For this review, take the finished solid that the model builds, in its own axes (mm). A direction names the side the tool comes from. Coordinates: 2 decimals unless noted, no trailing zeros. Loops run counter-clockwise (first coordinate to the right, second up) from the corner with the lowest first, then second, coordinate; pieces in that order, holes last. Notation, with made-up numbers: M -33,13 L -5,13 A21 cw -5,21 Z; hole C 51.5,64.25 d3. An arc over 180 degrees is marked long. Answer as a JSON object with one key per item and string values. Group by question number.
Item 1: Add section C-C (z = 16). State the section outline as (x, y) points (3 decimals).
Item 2: Add section A-A (x = 0). State the section outline as (y, z) points (1 decimal).
Item 3: Add section B-B (y = -0.5). State the section outline as (x, z) points (1 decimal).
Item 4: Wall thickness on L1, parallel to Y at x = 0, z = 14.3 (3 decimals); L2, parallel to Y at x = 0, z = 18.6 (3 decimals); L3, parallel to X at y = -2.25, z = 18.25: over which ranges is each line inside the solid? List them lowest first. Write a range as from..to.
Item 5: Add section D-D (y = -2). State the section outline as (x, z) points (1 decimal), then the cut area to 3 significant figures.
Item 6: Tool access review of faces 4 (the face through (2.731, 4.283, 18.545)), 5 (the face through (5.605, -0.098, 12.833)): name each direction out of +Z, -Z, +X, -X, +Y, -Y from which nothing blocks a thin tool from reaching the whole face with its end or side.
Item 7: Mouldability with a two-part tool opening along Y and no side actions: class faces 1 (the face through (0, -6.985, 16)), 2 (the face through (2, -2, 17.59)), 3 (the face through (-7.1, -0.1, 15.23)) as +Y half, -Y half, draft (parallel to the pull), parting line (faces both ways), or undercut.
Item 8: Insertion check: pin 1 (1.5 mm diameter, centred on y = -1.5, z = 18.5, fed in from +X); pin 2 (8 mm diameter, centred on x = -2, y = 0.5, fed in from +Z); pin 3 (5 mm diameter, centred on x = 1, y = 1.5, fed in from +Z). Each pin has a flat end and moves straight along its axis. Give the tip position at first contact, or say it passes through.
from build123d import *

# Parameters (mm, degrees)
F1_DEPTH = 6.985
F4_R     = 5.08
F5_DEPTH = 2.413
F6_R     = 2.54
F7_DEPTH = 5.2171329375
F8_R     = 1.27


with BuildPart() as f1:
    # F0 (on Front) → F1 (new body, symmetric)
    with BuildSketch(Plane.XZ):
        with BuildLine():
            ThreePointArc((-5.7697958184, 12.3733670625), (0, 13.6525), (5.7697958184, 12.3733670625))
            Line((5.7697958184, 12.3733670625), (8.4534217805, 18.1284215102))
            ThreePointArc((8.4534217805, 18.1284215102), (0, 20.0025), (-8.4534217805, 18.1284215102))
            Line((-8.4534217805, 18.1284215102), (-5.7697958184, 12.3733670625))
        make_face()
    extrude(amount=F1_DEPTH, both=True)

    # F4 (on plane+point) → F5 (cut)
    with BuildSketch(Plane.XY.offset(20.0025)):
        Circle(F4_R)
    extrude(amount=-F5_DEPTH, mode=Mode.SUBTRACT)

    # F6 (on face) → F7 (cut, through all)
    with BuildSketch(Plane.XY.offset(17.5895)):
        Circle(F6_R)
    extrude(amount=-F7_DEPTH, mode=Mode.SUBTRACT)

    # F8
    f8_edges = [f1.edges().sort_by_distance(p)[0] for p in [
        (8.453422, 0, 18.128422),
        (-8.453422, 0, 18.128422),
        (5.769796, 0, 12.373367),
        (-5.769796, 0, 12.373367),
    ]]
    fillet(f8_edges, radius=F8_R)


solid = f1.part
From the geometry:
{
 "1": {"outline": "M -7.461,-6.985 L 7.461,-6.985 L 7.461,6.985 L -7.461,6.985 Z; hole C 0,0 d5.08"},
 "2": {"outline": "M -7,13.7 L -2.5,13.7 L -2.5,17.6 L -5.1,17.6 L -5.1,20 L -7,20 Z; M 2.5,13.7 L 7,13.7 L 7,20 L 5.1,20 L 5.1,17.6 L 2.5,17.6 Z"},
 "3": {"outline": "M -7.9,16.9 L -6.3,13.5 A1.3 ccw -4.7,12.8 A13.7 cw -2.5,13.4 L -2.5,17.6 L -5.1,17.6 L -5.1,19.4 A20 ccw -7.2,18.7 A1.3 ccw Z; M 2.5,13.4 A13.7 cw 4.7,12.8 A1.3 ccw 6.3,13.5 L 7.9,16.9 A1.3 ccw 7.2,18.7 A20 ccw 5.1,19.4 L 5.1,17.6 L 2.5,17.6 Z"},
 "4": {"L1": "y = -6.985..-2.54, 2.54..6.985", "L2": "y = -6.985..-5.08, 5.08..6.985", "L3": "x = -7.75..-4.55, 4.55..7.75"},
 "5": {"outline": "M -7.9,16.9 L -6.3,13.5 A1.3 ccw -4.7,12.8 A13.7 cw -1.6,13.6 L -1.6,17.6 L -4.7,17.6 L -4.7,19.4 A20 ccw -7.2,18.7 A1.3 ccw Z; M 1.6,13.6 A13.7 cw 4.7,12.8 A1.3 ccw 6.3,13.5 L 7.9,16.9 A1.3 ccw 7.2,18.7 A20 ccw 4.7,19.4 L 4.7,17.6 L 1.6,17.6 Z", "area": "58.6 mm²"},
 "6": {"face 4": "+Z", "face 5": "-Z, +Y, -Y"},
 "7": {"face 1": "-Y half", "face 2": "undercut", "face 3": "draft"},
 "8": {"pin 1": "stops at x = 7.99", "pin 2": "stops at z = 19.86", "pin 3": "stops at z = 17.59"}
}
